The drawing under review shows one solid part. Ordinate dimensions are in mm from its lowest x, y, z. A direction names the side the tool comes from. Give positions to 0.01 mm unless a question says otherwise; leave off trailing zeros. Order: outer loops, then holes, each group sorted by start corner. A loop starts at its lowest first (then second) coordinate and runs counter-clockwise, first axis right, second up. Notation, with made-up numbers: (24.25, -34) -> (81.25, -34) arc R11 ccw to (81.25, -24) -> close; hole circle Ø6 at (-18.75, 71). An arc over 180 degrees is marked (long way). Return JSON: item names as keys, results as strings. Group by question number.
1) For the marked faces 1 and 2, list the 3-axis set-ups (+Z, -Z, +X, -X, +Y, -Y) from which the entire face can be reached by the end or side of a thin tool; tool diameter is ignored.
2) Add section A-A (x = 9.25). Give the boundary of the cut face in (y, z).
3) The part is to be moulded in two halves that separate along Z. For the marked faces 3, 4 and 5, say which applies: released by +Z, released by -Z, zero draft, split by the parting line, or undercut.
4) To check wall thickness, follow line 1 along Z through (x, y) = (6, 0.65); line 2 along Z through (x, y) = (13, 2.05); line 3 along X through (y, z) = (2.1, 6). State the ranges of each line that lie inside material, in increasing order.
5) Add section D-D (x = 12). Give the boundary of the cut face in (y, z).
6) Add section B-B (z = 8.5). Give the boundary of the cut face in (x, y), then the cut area to 3 significant figures.
7) Add section C-C (y = 3.75). Give the boundary of the cut face in (x, z).
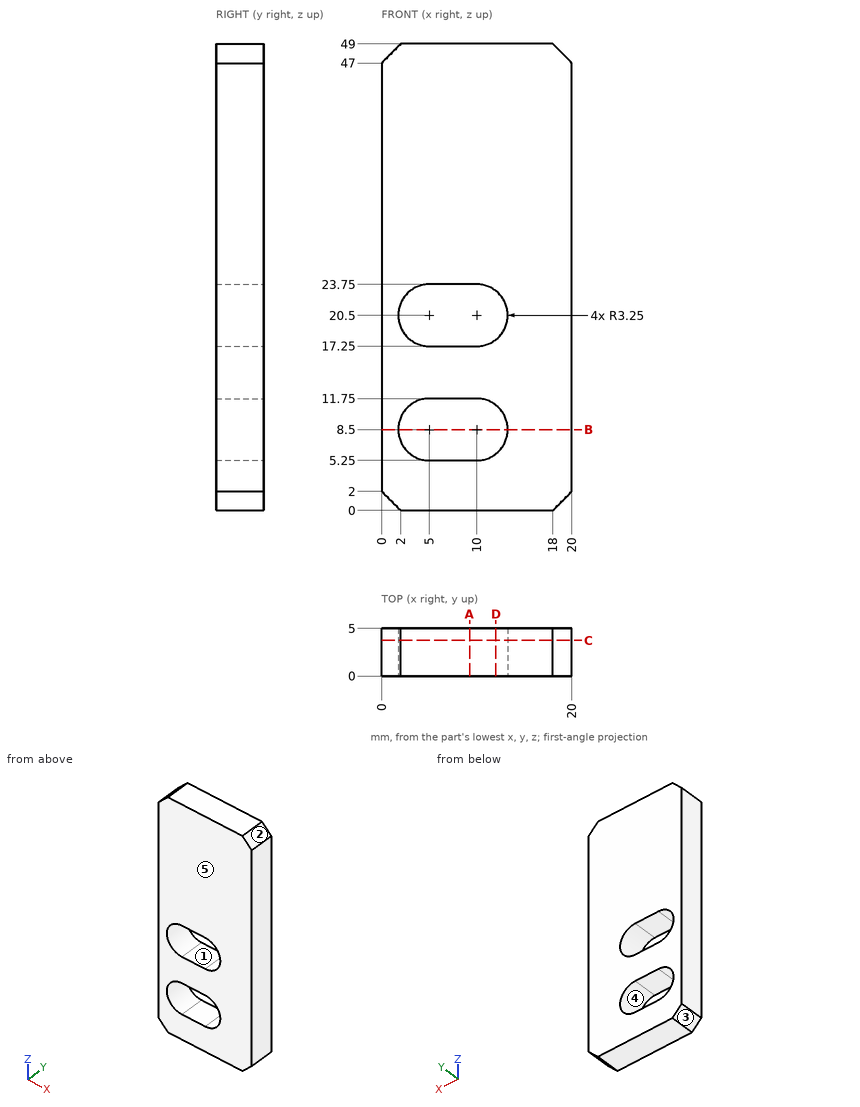
Evaluation:
{
 "1": {"face 1": "+Y, -Y", "face 2": "+Z, +X, +Y, -Y"},
 "2": {"outline": "(0, 0) -> (5, 0) -> (5, 5.25) -> (0, 5.25) -> close; (0, 11.75) -> (5, 11.75) -> (5, 17.25) -> (0, 17.25) -> close; (0, 23.75) -> (5, 23.75) -> (5, 49) -> (0, 49) -> close"},
 "3": {"face 3": "released by -Z", "face 4": "undercut", "face 5": "zero draft"},
 "4": {"line 1": "0 to 5.25, 11.75 to 17.25, 23.75 to 49", "line 2": "0 to 7.25, 9.75 to 19.25, 21.75 to 49", "line 3": "0 to 2.92, 12.08 to 20"},
 "5": {"outline": "(0, 0) -> (5, 0) -> (5, 5.94) -> (0, 5.94) -> close; (0, 11.06) -> (5, 11.06) -> (5, 17.94) -> (0, 17.94) -> close; (0, 23.06) -> (5, 23.06) -> (5, 49) -> (0, 49) -> close"},
 "6": {"outline": "(0, 0) -> (1.75, 0) -> (1.75, 5) -> (0, 5) -> close; (13.25, 0) -> (20, 0) -> (20, 5) -> (13.25, 5) -> close", "area": "42.5 mm^2"},
 "7": {"outline": "(0, 2) -> (2, 0) -> (18, 0) -> (20, 2) -> (20, 47) -> (18, 49) -> (2, 49) -> (0, 47) -> close; hole (5, 5.25) -> (10, 5.25) arc R3.25 ccw to (10, 11.75) -> (5, 11.75) arc R3.25 ccw to start; hole (5, 17.25) -> (10, 17.25) arc R3.25 ccw to (10, 23.75) -> (5, 23.75) arc R3.25 ccw to start"}
}
